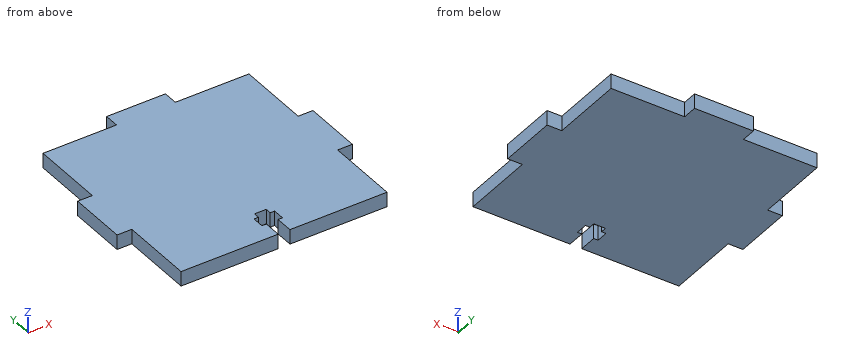
from build123d import *

# Parameters (mm, degrees)
BOSS_EXTRUDE1_DEPTH = 5
CUT_EXTRUDE1_DEPTH  = 10


with BuildPart() as part:
    # Sketch1 → Boss-Extrude1 (new body)
    with BuildSketch(Plane.XY):
        Polygon((-35, 35), (-10, 35), (-10, 40), (10, 40), (10, 35), (35, 35), (35, 10), (40, 10), (40, -10), (35, -10), (35, -35), (-35, -35), (-35, -10), (-40, -10), (-40, 10), (-35, 10), align=None)
    extrude(amount=BOSS_EXTRUDE1_DEPTH)

    # Sketch2 → Cut-Extrude1 (cut)
    with BuildSketch(Plane.XY.offset(5)):
        Polygon((-2, -35), (-2, -29), (-3.5, -29), (-3.5, -25), (-2, -25), (-2, -23), (2, -23), (2, -25), (3.5, -25), (3.5, -29), (2, -29), (2, -35), align=None)
    extrude(amount=-CUT_EXTRUDE1_DEPTH, mode=Mode.SUBTRACT)


solid = part.part
The listing builds one solid part. Answer for the finished solid, in the listing's coordinates (mm). Round coordinates to 2 decimals unless told otherwise and drop trailing zeros. Loops run counter-clockwise (first coordinate to the right, second up) from the corner with the lowest first, then second, coordinate; pieces in that order, holes last. Notation, with made-up numbers: M -23.75,-20.5 L 22.25,-20.5 A20 cw 22.25,-14.5 Z; hole C 7.5,-13.75 d9. An arc over 180 degrees is marked long. Write each question's results on one line, items separated by ' | '. Start each with the question number.
1) Each of these flat-tipped pins is pushed along its axis until it touches: pin 1 (2 mm diameter, centred on y = -24.5, z = 1.5, fed in from -X); pin 2 (1.5 mm diameter, centred on y = -19.5, z = 1.5, fed in from +X); pin 3 (3 mm diameter, centred on x = 25.5, z = 2.5, fed in from +Y). Where does it stop, or does it pass through?
2) Straight lines are drawn through the part: probe 1 along X at (y, z) = (17, 1); probe 2 along X at (y, z) = (-32, 0.45). For each, find the intervals that lie inside material, in ascending order.
3) Find section A-A on y = -27.5. Write down the section's boundary in (x, z), plus the area to 3 significant figures.
4) Find section B-B on z = 3.35. Write down the section's boundary in (x, y).
5) Find section C-C on x = -32. Write down the section's boundary in (y, z), plus the area to 3 significant figures.
Final values:
1) pin 1: x = -35 | pin 2: x = 35 | pin 3: y = 35
2) probe 1: -35 to 35 | probe 2: -35 to -2, 2 to 35
3) outline: M -35,0 L -3.5,0 L -3.5,5 L -35,5 Z; M 3.5,0 L 35,0 L 35,5 L 3.5,5 Z | area: 315 mm²
4) outline: M -40,-10 L -35,-10 L -35,-35 L -2,-35 L -2,-29 L -3.5,-29 L -3.5,-25 L -2,-25 L -2,-23 L 2,-23 L 2,-25 L 3.5,-25 L 3.5,-29 L 2,-29 L 2,-35 L 35,-35 L 35,-10 L 40,-10 L 40,10 L 35,10 L 35,35 L 10,35 L 10,40 L -10,40 L -10,35 L -35,35 L -35,10 L -40,10 Z
5) outline: M -35,0 L 35,0 L 35,5 L -35,5 Z | area: 350 mm²
